Can you work these out from the model? Positions are in its coordinate system, mm. A direction names the side the tool comes from. Give positions to 0.01 mm unless a question says otherwise; leave off trailing zeros. Write each loop counter-clockwise with the first axis right and the second up, starting at its lowest first coordinate (ties: lowest second). Pieces come first, ordered by that corner, then holes.
1. If I drill on probe 1 along Y at (x, z) = (12, 0); probe 2 along Z at (x, y) = (-3, -1); probe 3 along Y at (x, z) = (-21.5, 0), over which ranges is the centre line in solid material (lowest first)?
2. On a 3-axis mill with a long thin cutter (end or side, diameter ignored), from which of +Z, -Z, +X, -X, +Y, -Y can I reach the whole of each face in a straight line? I mean faces 1 (the cylindrical face through (13.7, 39.48, -43.06)), 2 (the flat face through (-14.635, 58, -10)), 3 (the cylindrical face through (-2.583, -24.796, -5.506)). Say none if no direction works.
3. I'm going to push flat-ended pins straight in: pin 1 (12 mm diameter, centred on x = -6.5, z = -1.5, fed in from +Y); pin 2 (2 mm diameter, centred on y = -44.5, z = 51.5, fed in from -X); pin 3 (12 mm diameter, centred on x = -15, z = 0.5, fed in from -Y); pin 4 (1.5 mm diameter, centred on y = 46.5, z = -45.5, fed in from +X). Where does each tip first touch, or does it pass through?
4. Suppose I cut it at D-D (x = -17.5). Please give me the cut outline in (y, z).
5. Thinking about a two-plate mould opening in Z: for faces 4 (the flat face through (41.245, -19, -19)), 5 (the conical face through (40.847, -63.618, -14.127)), 6 (the cylindrical face through (2.611, 13.352, 42.397)), which applies, pulls with the +Z half, pulls with the -Z half, needs draft (parallel to the pull), parting line crosses it, or undercut?
6. Suppose I cut it at C-C (x = -5.5). Please give me the cut outline in (y, z).
7. Suppose I cut it at A-A (z = 0). Please give me the cut outline in (x, y).
```python
from build123d import *

# Parameters (mm, degrees)
F2_SIZE = 6.35


with BuildPart() as f1:
    # F0 (on Front) → F1 (revolve)
    with BuildSketch(Plane.XZ):
        Polygon((-47.655353, 25.4), (41.244647, 25.4), (41.244647, 44.45), (-34.955353, 44.45), (-34.955353, 64.77), (-14.635353, 64.77), (-14.635353, 58.42), (41.244647, 58.42), (41.244647, 71.12), (-47.655353, 71.12), align=None)
    revolve(axis=Axis((-3.749629, 0, 0), (-1, 0, 0)))

    # F2
    f2_edges = [f1.edges().sort_by_distance(p)[0] for p in [
        (41.244647, 0, -71.12),
        (-47.655353, 0, -71.12),
    ]]
    chamfer(f2_edges, length=F2_SIZE)


solid = f1.part
```
Checks:
1. probe 1: y = -71.12 to -58.42, -44.45 to -25.4, 25.4 to 44.45, 58.42 to 71.12
1. probe 2: z = -71.11 to -58.41, -44.44 to -25.38, 25.38 to 44.44, 58.41 to 71.11
1. probe 3: y = -71.12 to -64.77, -44.45 to -25.4, 25.4 to 44.45, 64.77 to 71.12
2. face 1: +X
2. face 2: none
2. face 3: +X, -X
3. pin 1: stops at y = 71.12
3. pin 2: stops at x = -45.36
3. pin 3: stops at y = -71.12
3. pin 4: stops at x = 41.24
4. outline: circle Ø142.24 at (0, 0); circle Ø88.9 at (0, 0); hole circle Ø129.54 at (0, 0); hole circle Ø50.8 at (0, 0)
5. face 4: needs draft
5. face 5: parting line crosses it
5. face 6: undercut
6. outline: circle Ø142.24 at (0, 0); circle Ø88.9 at (0, 0); hole circle Ø116.84 at (0, 0); hole circle Ø50.8 at (0, 0)
7. outline: (-47.66, -64.77) - (-41.31, -71.12) - (34.89, -71.12) - (41.24, -64.77) - (41.24, -58.42) - (-14.64, -58.42) - (-14.64, -64.77) - (-34.96, -64.77) - (-34.96, -44.45) - (41.24, -44.45) - (41.24, -25.4) - (-47.66, -25.4) - close; (-47.66, 25.4) - (41.24, 25.4) - (41.24, 44.45) - (-34.96, 44.45) - (-34.96, 64.77) - (-14.64, 64.77) - (-14.64, 58.42) - (41.24, 58.42) - (41.24, 64.77) - (34.89, 71.12) - (-41.31, 71.12) - (-47.66, 64.77) - close
